Read the model definition and answer for the solid it produces. Units are mm, in the model's axes. Face numbers are marked on the shaded views. Coordinates: 2 decimals unless noted, no trailing zeros. Loops run counter-clockwise (first coordinate to the right, second up) from the corner with the lowest first, then second, coordinate; pieces in that order, holes last. Notation, with made-up numbers: (39.25, 1.5) -> (69.25, 1.5) arc R10 ccw to (69.25, 11.5) -> close; hole circle Ø1 at (72.5, 56.5). An arc over 180 degrees is marked (long way). Answer in a Markdown table with one row per item.
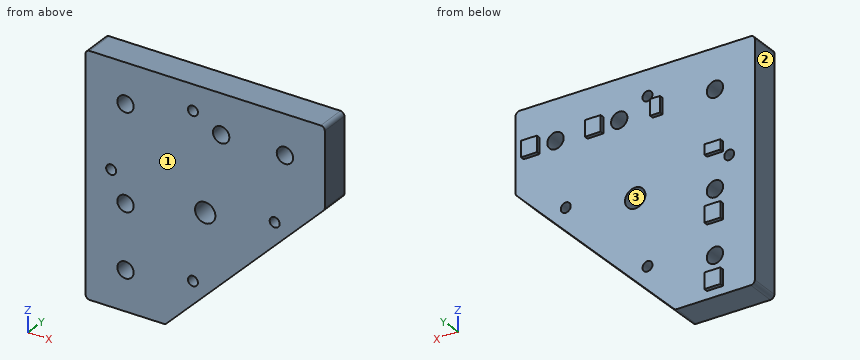
```python
from build123d import *

# Parameters (mm, degrees)
EXTRUDE_1_DEPTH             = 15
HOLE_WIZARD_M121_D          = 10.2
HOLE_WIZARD_M121_DEPTH      = 15
HOLE_WIZARD_M62_D           = 5
HOLE_WIZARD_M62_DEPTH       = 15
HOLE_WIZARD_8_2_8_2_1_D     = 8.2
HOLE_WIZARD_8_2_8_2_1_DEPTH = 15
SKETCH_9_W                  = 8
SKETCH_9_H                  = 8
SKETCH_9_H_2                = 5
SKETCH_9_W_2                = 5
EXTRUDE_2_DEPTH             = 2
FILLET_1_R                  = 2


with BuildPart() as part:
    # Эскиз1 → Бобышка-Вытянуть1 (new body)
    with BuildSketch(Plane(origin=(0, 0, 0), x_dir=(1, 0, 0), z_dir=(0, 1, 0))):
        Polygon((0, 0), (0, 120), (40, 120), (120, 40), (120, 0), align=None)
    extrude(amount=EXTRUDE_1_DEPTH)

    # Отверстие обработанное метчиком M121
    with Locations(Plane(origin=(0, 15, 0), x_dir=(1, 0, 0), z_dir=(0, 1, 0))):
        with Locations((60, 60)):
            Hole(HOLE_WIZARD_M121_D / 2, depth=HOLE_WIZARD_M121_DEPTH)

    # Отверстие обработанное метчиком M62
    with Locations(Plane(origin=(0, 15, 0), x_dir=(1, 0, 0), z_dir=(0, 1, 0))):
        with Locations((53.837049096, 94.849242405), (94.849242405, 53.837049096), (53.837049096, 12.824855787), (12.824855787, 53.837049096)):
            Hole(HOLE_WIZARD_M62_D / 2, depth=HOLE_WIZARD_M62_DEPTH)

    # Диаметр отверстия Ø8.2 (8.2)1
    with Locations(Plane(origin=(0, 15, 0), x_dir=(1, 0, 0), z_dir=(0, 1, 0))):
        with Locations((20, 100), (20, 68), (20, 20), (68, 20), (100, 20)):
            Hole(HOLE_WIZARD_8_2_8_2_1_D / 2, depth=HOLE_WIZARD_8_2_8_2_1_DEPTH)

    # Эскиз9 → Бобышка-Вытянуть2 (add)
    with BuildSketch(Plane(origin=(0, 15, 0), x_dir=(1, 0, 0), z_dir=(0, 1, 0))):
        with Locations((20, 112)):
            Rectangle(SKETCH_9_W, SKETCH_9_H)
        with Locations((20, 80)):
            Rectangle(SKETCH_9_W, SKETCH_9_H)
        with Locations((20, 48.75)):
            Rectangle(SKETCH_9_W, SKETCH_9_H_2)
        with Locations((48.75, 20)):
            Rectangle(SKETCH_9_W_2, SKETCH_9_H)
        with Locations((80, 20)):
            Rectangle(SKETCH_9_W, SKETCH_9_H)
        with Locations((112, 20)):
            Rectangle(SKETCH_9_W, SKETCH_9_H)
    extrude(amount=EXTRUDE_2_DEPTH)

    # Скругление1
    fillet_1_edges = [part.edges().sort_by_distance(p)[0] for p in [
        (0, 7.5, 0),
        (0, 7.5, -120),
        (40, 7.5, -120),
        (120, 7.5, -40),
        (120, 7.5, 0),
    ]]
    fillet(fillet_1_edges, radius=FILLET_1_R)


solid = part.part
```
1. Find the intervals of material crossed by probe 1 along X at (y, z) = (8.25, -20); probe 2 along Y at (x, z) = (91.5, -11); probe 3 along X at (y, z) = (6.5, -100), in increasing order.
A:
| item | result |
|---|---|
| probe 1 | x = 0 to 15.9, 24.1 to 63.9, 72.1 to 95.9, 104.1 to 120 |
| probe 2 | y = 0 to 15 |
| probe 3 | x = 0 to 15.9, 24.1 to 60 |
2. Given pin 1 Ø2 at (x, y) = (78.5, 16.5) entering from -Z; pin 2 Ø1 at (y, z) = (16.5, -82) entering from -X; pin 3 Ø2 at (y, z) = (16.5, -22) entering from +X; pin 4 Ø3 at (x, z) = (53.84, -12.82) entering from -Y, each flat-ended and moving along its own axis, determine where each tip first touches the part or whether it passes through.
A:
| item | result |
|---|---|
| pin 1 | stops at z = -24 |
| pin 2 | stops at x = 16 |
| pin 3 | stops at x = 116 |
| pin 4 | passes through |
3. The mould has two halves that part along X. Classify the marked faces 1, 2 and 3: pulls with the +X half, pulls with the -X half, needs draft (parallel to the pull), parting line crosses it, or undercut.
A:
| item | result |
|---|---|
| face 1 | needs draft |
| face 2 | pulls with the -X half |
| face 3 | undercut |
4. A cutting plane is placed at C-C on y = 1.5. Count the separate pieces of the cut face and the enclosed holes in it, and give its area (3 significant figures).
A:
| item | result |
|---|---|
| separate pieces | 1 |
| enclosed holes | 10 |
| area | 10,800 mm2 |
5. A cutting plane is placed at A-A on x = 68. Give the vertices of the cut face in (y, z).
A:
| item | result |
|---|---|
| outline | (0, -92) -> (15, -92) -> (15, -24.1) -> (0, -24.1) -> close; (0, -15.9) -> (15, -15.9) -> (15, 0) -> (0, 0) -> close |
6. A cutting plane is placed at B-B on z = -100. Give the vertices of the cut face in (x, y).
A:
| item | result |
|---|---|
| outline | (0, 0) -> (15.9, 0) -> (15.9, 15) -> (0, 15) -> close; (24.1, 0) -> (60, 0) -> (60, 15) -> (24.1, 15) -> close |
7. A cutting plane is placed at D-D on z = -81. Give the vertices of the cut face in (x, y).
A:
| item | result |
|---|---|
| outline | (0, 0) -> (79, 0) -> (79, 15) -> (24, 15) -> (24, 17) -> (16, 17) -> (16, 15) -> (0, 15) -> close |
